Model file for the job. Use its own axes, mm. A direction names the side the tool comes from. Round coordinates to 2 decimals unless told otherwise and drop trailing zeros. Order: outer loops, then holes, each group sorted by start corner. A loop starts at its lowest first (then second) coordinate and runs counter-clockwise, first axis right, second up. Notation, with made-up numbers: (25.25, 62.5) -> (45.25, 62.5) arc R26 ccw to (45.25, 98.5) -> close; hole circle Ø11 at (19.5, -38.5). An arc over 180 degrees is marked (long way). Use CSV: the item, a comma, the result in double quotes.
```python
from build123d import *

# Parameters (mm, degrees)
CROQUIS1_W                 = 73.5
CROQUIS1_H                 = 52.5
SALIENTE_EXTRUIR1_DEPTH    = 24
CORTAR_EXTRUIR1_START      = 24
CROQUIS4_W                 = 69.5
CROQUIS4_H                 = 48.5
CORTAR_EXTRUIR1_DEPTH      = 23
CORTAR_EXTRUIR4_START      = 24
CROQUIS5_W                 = 34.25
CROQUIS5_H                 = 23.75
CORTAR_EXTRUIR4_DEPTH      = 23
REDONDEO2_R                = 5
REDONDEO3_R                = 5
REDONDEO4_R                = 5
REDONDEO5_R                = 5
CORTAR_EXTRUIR5_DEPTH      = 52.143181364
CORTAR_EXTRUIR5_DEPTH_BACK = 52.143181364
CROQUIS6_W                 = 43.5
CROQUIS6_H                 = 32.5


with BuildPart() as part:
    # Croquis1 → Saliente-Extruir1 (new body)
    with BuildSketch(Plane(origin=(0, 0, 0), x_dir=(1, 0, 0), z_dir=(0, 1, 0))):
        Rectangle(CROQUIS1_W, CROQUIS1_H)
    extrude(amount=SALIENTE_EXTRUIR1_DEPTH)

    # Croquis4 → Cortar-Extruir1 (cut)
    with BuildSketch(Plane(origin=(0, 0, 0), x_dir=(1, 0, 0), z_dir=(0, 1, 0)).offset(CORTAR_EXTRUIR1_START)):
        Rectangle(CROQUIS4_W, CROQUIS4_H)
    extrude(amount=-CORTAR_EXTRUIR1_DEPTH, mode=Mode.SUBTRACT)

    # Croquis5 → Cortar-Extruir4 (cut)
    with BuildSketch(Plane(origin=(0, 0, 0), x_dir=(1, 0, 0), z_dir=(0, 1, 0)).offset(CORTAR_EXTRUIR4_START)):
        with Locations((19.625, 14.375)):
            Rectangle(CROQUIS5_W, CROQUIS5_H)
        with Locations((-19.625, 14.375)):
            Rectangle(CROQUIS5_W, CROQUIS5_H)
        with Locations((-19.625, -14.375)):
            Rectangle(CROQUIS5_W, CROQUIS5_H)
        with Locations((19.625, -14.375)):
            Rectangle(CROQUIS5_W, CROQUIS5_H)
    extrude(amount=-CORTAR_EXTRUIR4_DEPTH, mode=Mode.SUBTRACT)

    # Redondeo2
    redondeo2_edges = [part.edges().sort_by_distance(p)[0] for p in [
        (0, 1, -24.25),
    ]]
    fillet(redondeo2_edges, radius=REDONDEO2_R)

    # Redondeo3
    redondeo3_edges = [part.edges().sort_by_distance(p)[0] for p in [
        (-34.75, 1, 0),
    ]]
    fillet(redondeo3_edges, radius=REDONDEO3_R)

    # Redondeo4
    redondeo4_edges = [part.edges().sort_by_distance(p)[0] for p in [
        (0, 1, 24.25),
    ]]
    fillet(redondeo4_edges, radius=REDONDEO4_R)

    # Redondeo5
    redondeo5_edges = [part.edges().sort_by_distance(p)[0] for p in [
        (34.75, 1, 0),
    ]]
    fillet(redondeo5_edges, radius=REDONDEO5_R)

    # Croquis6 → Cortar-Extruir5 (cut, two sides: drawn at the far end of the back side and taken through both)
    with BuildSketch(Plane(origin=(0, 0, 0), x_dir=(1, 0, 0), z_dir=(0, 1, 0)).offset(-CORTAR_EXTRUIR5_DEPTH_BACK)):
        Rectangle(CROQUIS6_W, CROQUIS6_H)
    extrude(amount=CORTAR_EXTRUIR5_DEPTH + CORTAR_EXTRUIR5_DEPTH_BACK, mode=Mode.SUBTRACT)


solid = part.part
```
Q1. Cut at C-C (x = 15.5). Give the cut face in (y, z).
From the geometry:
outline,"(0, -26.25) -> (1, -26.25) -> (1, -16.25) -> (0, -16.25) -> close; (0, 16.25) -> (1, 16.25) -> (1, 26.25) -> (0, 26.25) -> close"
Q2. Cut at D-D (z = -20). Give the cut face in (x, y).
From the geometry:
outline,"(-36.75, 0) -> (36.75, 0) -> (36.75, 1) -> (2.5, 1) -> (2.5, 1.06) -> (-2.5, 1.06) -> (-2.5, 1) -> (-36.75, 1) -> close"
Q3. Pin check, flat tips, straight feed: pin 1 (2 mm diameter, centred on x = -33.5, y = 13.5, fed in from -Z); pin 2 (7.5 mm diameter, centred on y = 14, z = -22.5, fed in from -X); pin 3 (5.5 mm diameter, centred on x = 34, y = 7.5, fed in from +Z); pin 4 (7.5 mm diameter, centred on y = 12, z = -22.5, fed in from +X). Stop position of each tip, or through.
From the geometry:
pin 1,"passes through"
pin 2,"stops at x = -2.5"
pin 3,"stops at z = 2.5"
pin 4,"stops at x = 2.5"
Q4. Cut at B-B (y = 12.5). Give the cut face in (x, z), plus the area to 3 significant figures.
From the geometry:
outline,"(-36.75, -2.5) -> (-34.75, -2.5) -> (-34.75, 2.5) -> (-36.75, 2.5) -> close; (-2.5, -26.25) -> (2.5, -26.25) -> (2.5, -24.25) -> (-2.5, -24.25) -> close; (-2.5, 24.25) -> (2.5, 24.25) -> (2.5, 26.25) -> (-2.5, 26.25) -> close; (34.75, -2.5) -> (36.75, -2.5) -> (36.75, 2.5) -> (34.75, 2.5) -> close"
area,"40.0 mm²"
Q5. Which spindle directions (+Z, -Z, +X, -X, +Y, -Y) get a long thin tool onto all of the face, cutting with end or side? Do faces 1 (the flat face through (-1, 1, 17)), 2 (the flat face through (0, 15, 24.25)), 3 (the flat face through (-2.5, 12, 26)). Say none if no direction does.
From the geometry:
face 1,"+Y"
face 2,"+X, -X, +Y"
face 3,"+Z, -Z, -X, +Y"
Q6. Probe line 1 along X through (y, z) = (21, 1.5); line 2 along Y through (x, z) = (25, 7); line 3 along X through (y, z) = (5.5, 1). List the from-to ranges inside material, lowest first.
From the geometry:
line 1,"x = -36.75 to -34.75, 34.75 to 36.75"
line 2,"y = 0 to 1"
line 3,"x = -36.75 to -34.72, 34.72 to 36.75"
Q7. Mould opens along Z. For faces 4 (the cylindrical face through (0.04, 2.43, 22.75)), 5 (the cylindrical face through (-33.25, 2.43, -0.04)), 6 (the flat face through (0, 7, 26.25)), 7 (the flat face through (36, 12, -2.5)) say: +Z half, -Z half, draft (parallel to the pull), parting line (faces both ways), or undercut.
From the geometry:
face 4,"undercut"
face 5,"draft"
face 6,"+Z half"
face 7,"-Z half"
Q8. Cut at A-A (z = -10). Give the cut face in (x, y), plus the area to 3 significant figures.
From the geometry:
outline,"(-36.75, 0) -> (-21.75, 0) -> (-21.75, 1) -> (-36.75, 1) -> close; (21.75, 0) -> (36.75, 0) -> (36.75, 1) -> (21.75, 1) -> close"
area,"30.0 mm²"
